Geometry: see drawing. Coordinates: mm, zero at the bounding-box minimum. A direction names the side the tool comes from. Give positions to 0.01 mm unless a question says otherwise; leave off trailing zeros. Loops run counter-clockwise (first coordinate to the right, second up) from the corner with the lowest first, then second, coordinate; pieces in that order, holes last. Notation, with made-up numbers: M 15.25,87 L 30.25,87 A19 ccw 30.25,102 Z; hole C 4.5,71 d8. An arc over 180 degrees is marked long. Put each result on its own line as item: value.
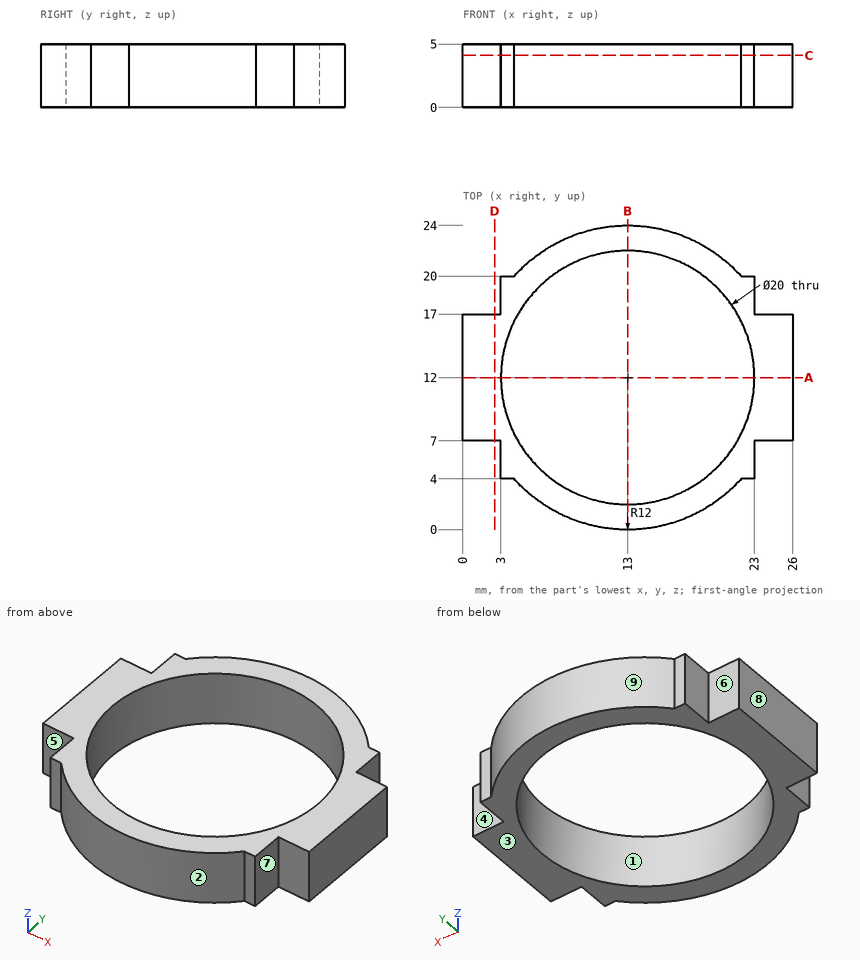
Item 1: Mould query, pull axis Y, two halves, no side actions, for the marked faces 1, 2, 3 and 4. Classes: pulls with the +Y half, pulls with the -Y half, needs draft (parallel to the pull), parting line crosses it, or undercut.
Output values:
face 1: undercut
face 2: pulls with the -Y half
face 3: needs draft
face 4: pulls with the +Y half
Item 2: Section B-B on x = 13. Output: boundary loops of the cut face in (y, z).
Output values:
outline: M 0,0 L 2,0 L 2,5 L 0,5 Z; M 22,0 L 24,0 L 24,5 L 22,5 Z
Item 3: Section D-D on x = 2.5. Output: boundary loops of the cut face in (y, z), then the cut area to 3 significant figures.
Output values:
outline: M 7,0 L 17,0 L 17,5 L 7,5 Z
area: 50.0 mm²
Item 4: Section A-A on y = 12. Output: boundary loops of the cut face in (x, z).
Output values:
outline: M 0,0 L 3,0 L 3,5 L 0,5 Z; M 23,0 L 26,0 L 26,5 L 23,5 Z
Item 5: Section C-C on z = 4.1. Output: boundary loops of the cut face in (x, y).
Output values:
outline: M 0,7 L 3,7 L 3,4 L 4.06,4 A12 ccw 21.94,4 L 23,4 L 23,7 L 26,7 L 26,17 L 23,17 L 23,20 L 21.94,20 A12 ccw 4.06,20 L 3,20 L 3,17 L 0,17 Z; hole C 13,12 d20
Item 6: Line query: probe 1 along Y at (x, z) = (13, 3.95); probe 2 along Y at (x, z) = (24, 4.45); probe 3 along Y at (x, z) = (20.5, 0.8). Output: solid intervals per line, ascending. Write a range as [from, to].
Output values:
probe 1: [0, 2], [22, 24]
probe 2: [7, 17]
probe 3: [2.63, 5.39], [18.61, 21.37]
Item 7: Pin query (flat end, axial travel): pin 1 Ø0.5 at (x, z) = (22.5, 2) entering from -Y; pin 2 Ø1.5 at (x, z) = (24.5, 2.5) entering from -Y; pin 3 Ø1.5 at (x, z) = (1.5, 2.5) entering from +Y. Return the tip coordinate at first contact, or that it passes through.
Output values:
pin 1: y = 4
pin 2: y = 7
pin 3: y = 17
Item 8: Set-up query: the marked faces 5, 6, 7, 8 and 9. Return all of +Z, -Z, +X, -X, +Y, -Y with unobstructed straight access to the full face (end or side cutting, diameter ignored); none if empty.
Output values:
face 5: +Z, -Z, -X, -Y
face 6: +Z, -Z, -X, +Y
face 7: +Z, -Z, +X, -Y
face 8: +Z, -Z, -X, +Y, -Y
face 9: +Z, -Z, +Y
